Geometry: final body of the model. Coordinates: model frame, mm. Face numbers are marked on the shaded views. A direction names the side the tool comes from. Give positions to 0.01 mm unless a question says otherwise; leave off trailing zeros. Order: outer loops, then holes, each group sorted by start corner. A loop starts at its lowest first (then second) coordinate and runs counter-clockwise, first axis right, second up. Notation, with made-up numbers: (84.25, -30.75) - (110.25, -30.75) arc R25 ccw to (110.25, 0.25) - close; hole circle Ø2 at (68.25, 14.25). An arc over 180 degrees is marked (long way). One line per item, written item: value.
```python
from build123d import *

# Parameters (mm, degrees)
F0_W     = 3.9
F0_H     = 5.8
F0_W_2   = 1.9
F0_H_2   = 2
F2_R     = 4.166667
F3_DEPTH = 6


with BuildPart() as f1:
    # F0 (on Front) → F1 (revolve)
    with BuildSketch(Plane.XZ):
        Polygon((17.5, 17.3), (0, 17.3), (0, 12.3), (4.1, 12.3), (8, 12.3), (17.5, 12.3), align=None)
        with Locations((6.05, 9.4)):
            Rectangle(F0_W, F0_H)
        Polygon((8, 6.5), (4.1, 6.5), (4.1, 2), (6, 2), (11.9, 2), (11.9, 6.5), align=None)
        with Locations((5.05, 1)):
            Rectangle(F0_W_2, F0_H_2)
    revolve(axis=Axis((0, 0, 14.8), (0, 0, -1)))

    # F2 (on face) → F3 (join)
    with BuildSketch(Plane(origin=(0, 0, 12.3), x_dir=(1, 0, 0), z_dir=(0, 0, -1))):
        with BuildLine():
            ThreePointArc((-8, -5), (0, -8), (8, -5))
            Line((8, -5), (8, 5))
            ThreePointArc((8, 5), (0, 8), (-8, 5))
            Line((-8, 5), (-8, -5))
        make_face()
        Circle(F2_R, mode=Mode.SUBTRACT)
    extrude(amount=F3_DEPTH)


solid = f1.part
```
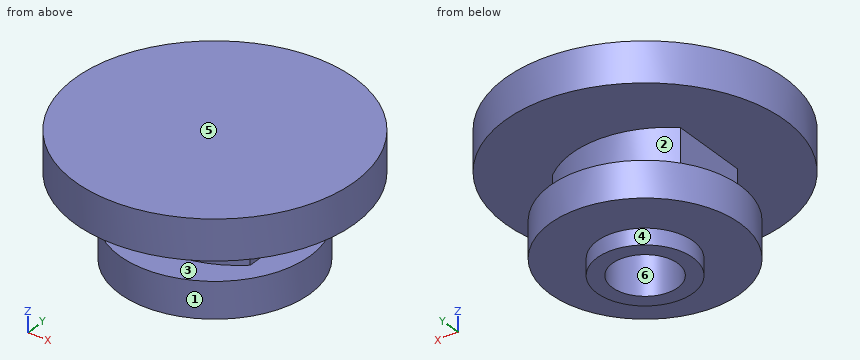
1) Section C-C, the plane x = 0. Return loops of the section in (y, z), then the cut area to 3 significant figures.
Answers below:
outline: (-17.5, 12.3) - (-8, 12.3) - (-8, 6.5) - (-11.9, 6.5) - (-11.9, 2) - (-6, 2) - (-6, 0) - (-4.1, 0) - (-4.1, 12.3) - (4.1, 12.3) - (4.1, 0) - (6, 0) - (6, 2) - (11.9, 2) - (11.9, 6.5) - (8, 6.5) - (8, 12.3) - (17.5, 12.3) - (17.5, 17.3) - (-17.5, 17.3) - close
area: 298 mm^2
2) Section A-A, the plane z = 11.25. Return loops of the section in (x, y).
Answers below:
outline: (-8, -5) arc R12.17 ccw to (8, -5) - (8, 5) arc R12.17 ccw to (-8, 5) - close; hole circle Ø8.2 at (0, 0)
3) Material intervals for line 1 along X through (y, z) = (0, 6); line 2 along Z through (x, y) = (-5.5, -7), sorted ascending.
Answers below:
line 1: -11.9 to -4.1, 4.1 to 11.9
line 2: 2 to 6.5, 12.3 to 17.3
4) Section B-B, the plane y = 8.5. Return loops of the section in (x, z).
Answers below:
outline: (-15.3, 12.3) - (15.3, 12.3) - (15.3, 17.3) - (-15.3, 17.3) - close; (-8.33, 2) - (8.33, 2) - (8.33, 6.5) - (-8.33, 6.5) - close
5) Mould query, pull axis X, two halves, no side actions, for the marked faces 4, 5 and 6. Classes: released by +X, released by -X, zero draft, split by the parting line, or undercut.
Answers below:
face 4: split by the parting line
face 5: zero draft
face 6: undercut
6) Set-up query: the marked faces 1, 2 and 3. Return all of +Z, -Z, +X, -X, +Y, -Y with unobstructed straight access to the full face (end or side cutting, diameter ignored); none if empty.
Answers below:
face 1: -Z
face 2: +Y
face 3: none
7) First-contact query: pin 1 (5 mm diameter, centred on x = -11, z = 11.5, fed in from -Y); pin 2 (6 mm diameter, centred on x = 4, z = 6, fed in from +Y); pin 3 (8 mm diameter, centred on y = 6.5, z = 13.5, fed in from -X); pin 4 (17.5 mm diameter, centred on x = -1, y = -2.5, fed in from -Z). Flat tips, straight axial feed; report the tip coordinate or a pass-through.
Answers below:
pin 1: y = -15.22
pin 2: y = 11.86
pin 3: x = -17.32
pin 4: z = 0
